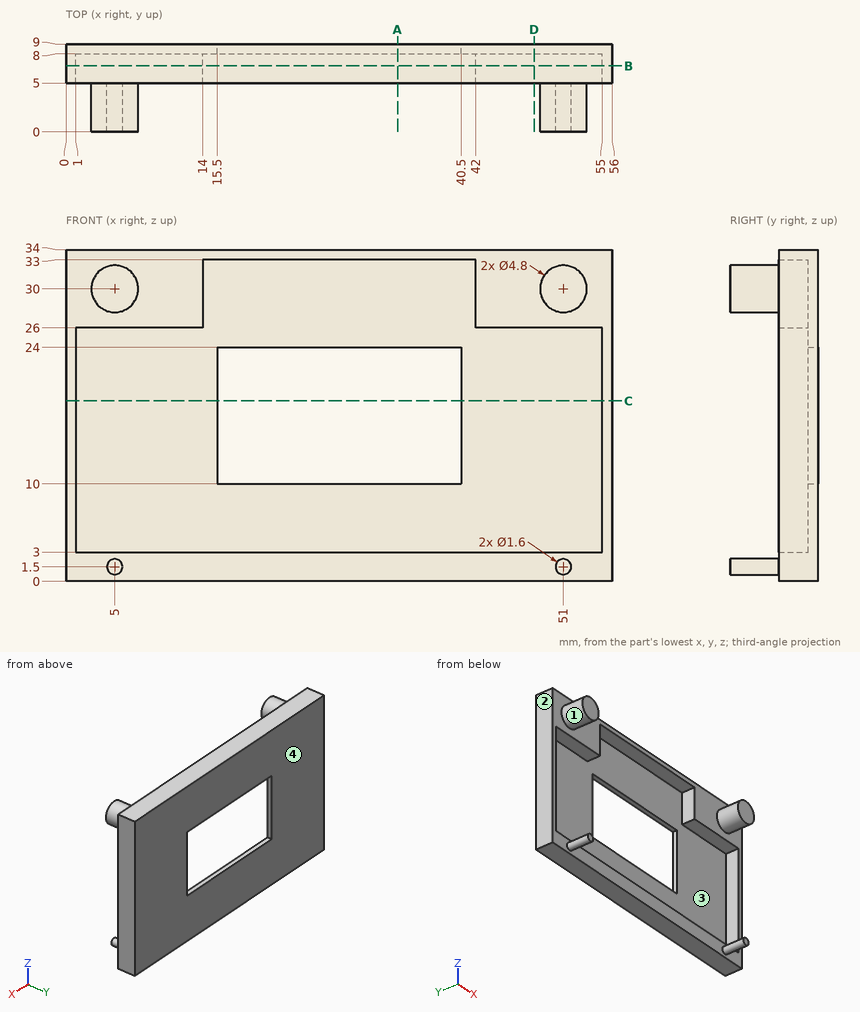
The drawing under review shows one solid part. Ordinate dimensions are in mm from its lowest x, y, z. A direction names the side the tool comes from. Give positions to 0.01 mm unless a question says otherwise; leave off trailing zeros. Loops run counter-clockwise (first coordinate to the right, second up) from the corner with the lowest first, then second, coordinate; pieces in that order, holes last. Notation, with made-up numbers: M -40,23.25 L -29,23.25 A19 ccw -29,51.25 Z; hole C -37,63 d9. An arc over 180 degrees is marked long. Return JSON: item names as keys, results as strings. Group by question number.
Item 1: Tool access review of the marked faces 1 and 2: name each direction out of +Z, -Z, +X, -X, +Y, -Y from which nothing blocks a thin tool from reaching the whole face with its end or side.
Item 2: We need section A-A (x = 34). Give the boundary of the cut face in (y, z).
Item 3: We need section D-D (x = 48). Give the boundary of the cut face in (y, z), and give its area (3 significant figures).
Item 4: We need section C-C (z = 18.5). Give the boundary of the cut face in (x, y), and give its area (3 significant figures).
Item 5: For probe 1 along Z at (x, y) = (52, 7.75); probe 2 along Z at (x, y) = (16.5, 7); probe 3 along Y at (x, z) = (51.5, 27.5), list the stretches that pass through material, from the lowest coordinate up.
Item 6: We need section B-B (y = 6.75). Give the boundary of the cut face in (x, z).
Item 7: Mouldability with a two-part tool opening along Z and no side actions: class the marked faces 3 and 4 as released by +Z, released by -Z, zero draft, split by the parting line, or undercut.
Item 8: Insertion check: pin 1 Ø3.5 at (x, y) = (28, 7) entering from -Z; pin 2 Ø10 at (x, z) = (38, 28) entering from -Y; pin 3 Ø15 at (x, z) = (21.5, 25) entering from -Y. Each pin has a flat end and moves straight along its axis. Give the tip position at first contact, or say it passes through.
Output:
{
 "1": {"face 1": "-Y", "face 2": "+Z, -Z, -X, +Y, -Y"},
 "2": {"outline": "M 5,0 L 9,0 L 9,10 L 8,10 L 8,3 L 5,3 Z; M 5,33 L 8,33 L 8,24 L 9,24 L 9,34 L 5,34 Z"},
 "3": {"outline": "M 5,0 L 9,0 L 9,34 L 5,34 L 5,26 L 8,26 L 8,3 L 5,3 Z", "area": "67.0 mm^2"},
 "4": {"outline": "M 0,5 L 1,5 L 1,8 L 15.5,8 L 15.5,9 L 0,9 Z; M 40.5,8 L 55,8 L 55,5 L 56,5 L 56,9 L 40.5,9 Z", "area": "37.0 mm^2"},
 "5": {"probe 1": "z = 0 to 3, 26 to 34", "probe 2": "z = 0 to 3, 33 to 34", "probe 3": "y = 5 to 9"},
 "6": {"outline": "M 0,0 L 56,0 L 56,34 L 0,34 Z; hole M 1,3 L 55,3 L 55,26 L 42,26 L 42,33 L 14,33 L 14,26 L 1,26 Z"},
 "7": {"face 3": "undercut", "face 4": "zero draft"},
 "8": {"pin 1": "stops at z = 0", "pin 2": "stops at y = 5", "pin 3": "stops at y = 8"}
}
